CAD build for the part. Positions are in the model's coordinates, mm. A direction names the side the tool comes from. Round coordinates to 2 decimals unless told otherwise and drop trailing zeros. Write each loop counter-clockwise with the first axis right and the second up, starting at its lowest first coordinate (ties: lowest second). Pieces come first, ordered by that corner, then holes. Notation, with made-up numbers: (36, 24.25) - (45, 24.25) arc R20 ccw to (45, 30.25) - close; hole circle Ø6 at (18.5, 50). An arc over 180 degrees is marked (long way). Put each result on its own line as item: value. Start each with the question number.
Item 1: Mould opens along X. For faces 1 (the flat face through (45.432, 7.412, 21.337)), 2 (the flat face through (0, 17, 13)), 3 (the flat face through (30, 23, 0)), 4 (the flat face through (50, 4.75, 21)) say: released by +X, released by -X, zero draft, split by the parting line, or undercut.
Item 2: Drill centre lines: line 1 (Y direction, x = 50, z = 6.25); line 2 (X direction, y = 16, z = 20.5); line 3 (Y direction, x = 52, z = 9). Where is each one in solid material? Low to high. Write a range as from..to.
Item 3: Cut at C-C (y = 8.5). Give the cut face in (x, z), and give its area (3 significant figures).
Item 4: Cut at D-D (x = 31). Give the cut face in (y, z), and give its area (3 significant figures).
Item 5: Pin check, flat tips, straight feed: pin 1 Ø5 at (x, z) = (51, 13.5) entering from +Y; pin 2 Ø4 at (x, y) = (10, 35) entering from +Z; pin 3 Ø9 at (x, y) = (50, 35) entering from +Z; pin 4 Ø5.5 at (x, z) = (24.5, 20.5) entering from +Y. Stop position of each tip, or through.
Item 6: Cut at B-B (z = 3). Give the cut face in (x, y).
Item 7: 3-axis set-ups, long thin cutter, end or side, ignore diameter. For faces 5 (the cylindrical face through (34.83, 11.888, 7.883)), 6 (the flat face through (40, 30, 12)), 7 (the flat face through (28, 4, 10)), 8 (the flat face through (50, 40.25, 11)), 9 (the cylindrical face through (10.46, 38.47, 4.93)): which of +Z, -Z, +X, -X, +Y, -Y reach the whole face in a straight line?
Item 8: Cut at A-A (x = 50). Give the cut face in (y, z), and give its area (3 significant figures).
```python
from build123d import *

# Parameters (mm, degrees)
SKETCH1_W           = 60
SKETCH1_H           = 45
BOSS_EXTRUDE1_DEPTH = 35
SKETCH2_R           = 4.5
CUT_EXTRUDE1_DEPTH  = 50
SKETCH3_R           = 11.25
CUT_EXTRUDE2_DEPTH  = 4
SKETCH6_W           = 20
SKETCH6_H           = 25
CUT_EXTRUDE4_DEPTH  = 30
CUT_EXTRUDE3_DEPTH  = 80
SKETCH7_R           = 1.75
CUT_EXTRUDE5_DEPTH  = 25
SKETCH8_R           = 3.5
CUT_EXTRUDE6_DEPTH  = 44
CUT_EXTRUDE7_START  = 35
CUT_EXTRUDE7_DEPTH  = 25
SKETCH10_R          = 5.1
CUT_EXTRUDE8_DEPTH  = 10.5


with BuildPart() as part:
    # Sketch1 → Boss-Extrude1 (new body)
    with BuildSketch(Plane.XY):
        with Locations((30, 22.5)):
            Rectangle(SKETCH1_W, SKETCH1_H)
    extrude(amount=BOSS_EXTRUDE1_DEPTH)

    # Sketch2 → Cut-Extrude1 (cut)
    with BuildSketch(Plane.XZ):
        with Locations(Location((30, 15, 0), (0, 0, 270))):
            Circle(SKETCH2_R)
    extrude(amount=-CUT_EXTRUDE1_DEPTH, mode=Mode.SUBTRACT)

    # Sketch3 → Cut-Extrude2 (cut)
    with BuildSketch(Plane.XZ):
        with Locations(Location((30, 15, 0), (0, 0, 270))):
            Circle(SKETCH3_R)
    extrude(amount=-CUT_EXTRUDE2_DEPTH, mode=Mode.SUBTRACT)

    # Sketch6 → Cut-Extrude4 (cut)
    with BuildSketch(Plane.XY.offset(35)):
        with Locations((30, 32.5)):
            Rectangle(SKETCH6_W, SKETCH6_H)
    extrude(amount=-CUT_EXTRUDE4_DEPTH, mode=Mode.SUBTRACT)

    # Sketch4 → Cut-Extrude3 (cut)
    with BuildSketch(Plane(origin=(60, 0, 0), x_dir=(0, 0, -1), z_dir=(1, 0, 0))):
        Polygon((-35, 0), (-10, 45), (-35, 45), align=None)
    extrude(amount=-CUT_EXTRUDE3_DEPTH, mode=Mode.SUBTRACT)

    # Sketch7 → Cut-Extrude5 (cut)
    with BuildSketch(Plane.XZ.offset(-4)):
        with Locations(Location((24.5, 20.5, 0), (0, 0, 270))):
            Circle(SKETCH7_R)
        with Locations(Location((35.5, 20.5, 0), (0, 0, 270))):
            Circle(SKETCH7_R)
        with Locations(Location((35.5, 9.5, 0), (0, 0, 270))):
            Circle(SKETCH7_R)
        with Locations(Location((24.5, 9.5, 0), (0, 0, 270))):
            Circle(SKETCH7_R)
    extrude(amount=-CUT_EXTRUDE5_DEPTH, mode=Mode.SUBTRACT)

    # Sketch8 → Cut-Extrude6 (cut)
    with BuildSketch(Plane(origin=(0, 0, 0), x_dir=(-1, 0, 0), z_dir=(0, 0, -1))):
        with Locations((-50, 10)):
            Circle(SKETCH8_R)
        with Locations((-50, 35)):
            Circle(SKETCH8_R)
        with Locations((-10, 35)):
            Circle(SKETCH8_R)
        with Locations((-10, 10)):
            Circle(SKETCH8_R)
    extrude(amount=-CUT_EXTRUDE6_DEPTH, mode=Mode.SUBTRACT)

    # Sketch9 → Cut-Extrude7 (cut)
    with BuildSketch(Plane.XY.offset(CUT_EXTRUDE7_START)):
        Polygon((6.968911087, 40.25), (3.937822174, 35), (6.968911087, 29.75), (13.031088913, 29.75), (16.062177826, 35), (13.031088913, 40.25), align=None)
        Polygon((13.031088913, 4.75), (16.062177826, 10), (13.031088913, 15.25), (6.968911087, 15.25), (3.937822174, 10), (6.968911087, 4.75), align=None)
        Polygon((53.031088913, 29.75), (56.062177826, 35), (53.031088913, 40.25), (46.968911087, 40.25), (43.937822174, 35), (46.968911087, 29.75), align=None)
        Polygon((53.031088913, 4.75), (56.062177826, 10), (53.031088913, 15.25), (46.968911087, 15.25), (43.937822174, 10), (46.968911087, 4.75), align=None)
    extrude(amount=-CUT_EXTRUDE7_DEPTH, mode=Mode.SUBTRACT)

    # Sketch10 → Cut-Extrude8 (cut)
    with BuildSketch(Plane.XZ.offset(-4)):
        with Locations(Location((30, 15, 0), (0, 0, 270))):
            Circle(SKETCH10_R)
    extrude(amount=-CUT_EXTRUDE8_DEPTH, mode=Mode.SUBTRACT)


solid = part.part
```
Output values:
1. face 1: undercut
1. face 2: released by -X
1. face 3: zero draft
1. face 4: undercut
2. line 1: 0..6.5, 13.5..31.5, 38.5..45
2. line 2: 0..22.75, 26.25..33.75, 37.25..60
2. line 3: 0..7.13, 12.87..32.13, 37.87..45
3. outline: (0, 0) - (6.84, 0) - (6.84, 10) - (4.8, 10) - (4.8, 30.28) - (0, 30.28) - close; (13.16, 0) - (46.84, 0) - (46.84, 10) - (44.8, 10) - (44.8, 30.28) - (15.2, 30.28) - (15.2, 10) - (13.16, 10) - close; (53.16, 0) - (60, 0) - (60, 30.28) - (55.2, 30.28) - (55.2, 10) - (53.16, 10) - close; hole circle Ø3.5 at (24.5, 9.5); hole circle Ø3.5 at (24.5, 20.5); hole circle Ø10.2 at (30, 15); hole circle Ø3.5 at (35.5, 9.5); hole circle Ø3.5 at (35.5, 20.5)
3. area: 1,150 mm2
4. outline: (0, 0) - (45, 0) - (45, 5) - (20, 5) - (20, 10.61) - (14.5, 10.61) - (14.5, 10) - (4, 10) - (4, 3.79) - (0, 3.79) - close; (0, 26.21) - (4, 26.21) - (4, 20) - (14.5, 20) - (14.5, 19.39) - (20, 19.39) - (20, 23.89) - (0, 35) - close
4. area: 471 mm2
5. pin 1: y = 43.2
5. pin 2: through
5. pin 3: z = 10
5. pin 4: y = 20
6. outline: (0, 0) - (60, 0) - (60, 45) - (0, 45) - close; hole circle Ø7 at (10, 10); hole circle Ø7 at (10, 35); hole circle Ø7 at (50, 10); hole circle Ø7 at (50, 35)
7. face 5: +Y, -Y
7. face 6: +Z, +Y
7. face 7: -Y
7. face 8: +Z
7. face 9: +Z, -Z
8. outline: (0, 0) - (6.5, 0) - (6.5, 10) - (4.75, 10) - (4.75, 32.36) - (0, 35) - close; (13.5, 0) - (31.5, 0) - (31.5, 10) - (29.75, 10) - (29.75, 18.47) - (15.25, 26.53) - (15.25, 10) - (13.5, 10) - close; (38.5, 0) - (45, 0) - (45, 10) - (40.25, 12.64) - (40.25, 10) - (38.5, 10) - close
8. area: 610 mm2
